from build123d import *

# Parameters (mm, degrees)
SKETCH1_R                = 0.25
SKETCH1_W                = 17
SKETCH1_H                = 6
BOSS_EXTRUDE1_DEPTH      = 5
FILLET1_R                = 2
M2_5X0_45_TAPPED_HOLE1_D = 2.05
M3_CLEARANCE_HOLE1_D     = 3.4
M3_CLEARANCE_HOLE1_DEPTH = 3


with BuildPart() as part:
    # Sketch1 → Boss-Extrude1 (new body)
    with BuildSketch(Plane.XY):
        Polygon((-15, 0), (15, 0), (15, 18), (12.5, 20), (12.5, 32.461249695), (-12.5, 32.461249695), (-12.5, 20), (-15, 18), align=None)
        with Locations((-10.5, 30.461249695)):
            Circle(SKETCH1_R, mode=Mode.SUBTRACT)
        with Locations((-10.5, 17.961249695)):
            Circle(SKETCH1_R, mode=Mode.SUBTRACT)
        with Locations((10.5, 30.461249695)):
            Circle(SKETCH1_R, mode=Mode.SUBTRACT)
        with Locations((10.5, 17.961249695)):
            Circle(SKETCH1_R, mode=Mode.SUBTRACT)
        Polygon((-11, 15), (-8.5, 17), (-8.5, 19.461249695), (8.5, 19.461249695), (8.5, 17), (11, 15), (11, 3), (-11, 3), align=None, mode=Mode.SUBTRACT)
        with Locations((0, 25.461249695)):
            Rectangle(SKETCH1_W, SKETCH1_H, mode=Mode.SUBTRACT)
    extrude(amount=BOSS_EXTRUDE1_DEPTH)

    # Fillet1
    fillet1_edges = [part.edges().sort_by_distance(p)[0] for p in [
        (-15, 18, 2.5),
        (-12.5, 20, 2.5),
        (-12.5, 32.461249695, 2.5),
        (12.5, 32.461249695, 2.5),
        (12.5, 20, 2.5),
        (15, 18, 2.5),
        (-11, 15, 2.5),
        (11, 15, 2.5),
        (8.5, 17, 2.5),
        (-8.5, 17, 2.5),
    ]]
    fillet(fillet1_edges, radius=FILLET1_R)

    # M2.5x0.45 Tapped Hole1 (through all)
    with Locations(Plane.XY.offset(5)):
        with Locations((-10.5, 17.961249695), (10.5, 30.461249695), (10.5, 17.961249695), (-10.5, 30.461249695)):
            Hole(M2_5X0_45_TAPPED_HOLE1_D / 2)

    # M3 Clearance Hole1
    with Locations(Plane(origin=(0, 0, 0), x_dir=(-1, 0, 0), z_dir=(0, -1, 0))):
        with Locations((8, -2.5), (-8, -2.5)):
            Hole(M3_CLEARANCE_HOLE1_D / 2, depth=M3_CLEARANCE_HOLE1_DEPTH)


solid = part.part
Build history of the part. All positions in model axes, mm. A direction names the side the tool comes from. Give positions to 0.01 mm unless a question says otherwise; leave off trailing zeros. Loops run counter-clockwise (first coordinate to the right, second up) from the corner with the lowest first, then second, coordinate; pieces in that order, holes last. Notation, with made-up numbers: (27, 83.5) -> (56, 83.5) arc R14 cw to (56, 88.5) -> close; hole circle Ø5 at (-35, 29.25). An arc over 180 degrees is marked (long way). Answer in a Markdown table with one row per item.
Item 1: Slice it at A-A on x = 8. Write the cut outline in (y, z).
Findings below:
| item | result |
|---|---|
| outline | (0, 0) -> (3, 0) -> (3, 0.8) -> (0, 0.8) -> close; (0, 4.2) -> (3, 4.2) -> (3, 5) -> (0, 5) -> close; (19.46, 0) -> (22.46, 0) -> (22.46, 5) -> (19.46, 5) -> close; (28.46, 0) -> (32.46, 0) -> (32.46, 5) -> (28.46, 5) -> close |
Item 2: Mould opens along X. For faces 1 (the cylindrical face through (-10.28, 16.96, 2.46)), 2 (the flat face through (-12.5, 26, 2)), 3 (the flat face through (13.76, 18.99, 2.46)), 4 (the flat face through (0, 20, 5)) say: pulls with the +X half, pulls with the -X half, needs draft (parallel to the pull), parting line crosses it, or undercut.
Findings below:
| item | result |
|---|---|
| face 1 | undercut |
| face 2 | pulls with the -X half |
| face 3 | pulls with the +X half |
| face 4 | needs draft |
Item 3: Tool access for faces 5 (the flat face through (12.5, 26, 2)), 6 (the cylindrical face through (8.703, 17.084, 2.535)), 7 (the flat face through (0, 32.461, 2)): list every direction of +Z, -Z, +X, -X, +Y, -Y with a clear straight run to the whole face (end or side of a thin tool).
Findings below:
| item | result |
|---|---|
| face 5 | +Z, -Z, +X, +Y |
| face 6 | +Z, -Z |
| face 7 | +Z, -Z, +X, -X, +Y |
Item 4: Slice it at C-C on z = 2.5. Give the number of separate pieces and of enclosed holes in the cut face, plus the area to 3 significant figures.
Findings below:
| item | result |
|---|---|
| separate pieces | 2 |
| enclosed holes | 5 |
| area | 424 mm² |
Item 5: Probe line 1 along Y through (x, z) = (0.25, 3.05); line 2 along X through (y, z) = (27, 0.6); line 3 along Y through (x, z) = (10.5, 1.2). List the from-to ranges inside material, lowest first. Write a range as [from, to].
Findings below:
| item | result |
|---|---|
| line 1 | y = [0, 3], [19.46, 22.46], [28.46, 32.46] |
| line 2 | x = [-12.5, -8.5], [8.5, 12.5] |
| line 3 | y = [0, 3], [15.36, 16.94], [18.99, 29.44], [31.49, 32.46] |
Item 6: Flat gauge pins, fed straight in: P1, Ø1.8, axis at x = -10.5, y = 30.46, coming from the -Z side; P2, Ø1.2, axis at y = 19, z = 1.5, coming from the +X side; P3, Ø2, axis at x = -8, z = 2.5, coming from the -Y side; P4, Ø1.2, axis at y = 18.5, z = 2.5, coming from the -X side. Where does each tip first touch, or does it go through?
Findings below:
| item | result |
|---|---|
| P1 | passes through |
| P2 | stops at x = 14.47 |
| P3 | stops at y = 16.64 |
| P4 | stops at x = -14.81 |
Item 7: Slice it at B-B on y = 13. Write the cut outline in (x, z).
Findings below:
| item | result |
|---|---|
| outline | (-15, 0) -> (-11, 0) -> (-11, 5) -> (-15, 5) -> close; (11, 0) -> (15, 0) -> (15, 5) -> (11, 5) -> close |
